Part model, mm, in its own coordinate system. A direction names the side the tool comes from. Coordinates: 2 decimals unless noted, no trailing zeros. One line per question, with ' | ' between items. Start each with the question number.
from build123d import *

# Parameters (mm, degrees)
F0_R            = 45
F0_R_2          = 12.5
F1_DEPTH        = 5
F3_DEPTH        = 10.001
F3_COPIES_COUNT = 8
F4_SIZE         = 0.5
F5_R            = 2


# Not quite as in the source:
# - a pattern or mirror of a feature is missing from the dataset's text; its kind, count and spacing are read off the source's solid


with BuildPart() as f1:
    # F0 (on Front) → F1 (new body, symmetric)
    with BuildSketch(Plane.XZ):
        Circle(F0_R)
        Circle(F0_R_2, mode=Mode.SUBTRACT)
    extrude(amount=F1_DEPTH, both=True)

    # F2 (on face) → F3 (cut, through all)
    with BuildSketch(Plane.XZ.offset(5)):
        Polygon((3.36, 28.75), (0, 33.55), (-3.36, 28.75), (0, 23.95), align=None)
    f3 = extrude(amount=-F3_DEPTH, mode=Mode.SUBTRACT)

    # F3_copies: F3 ×8 about axis
    f3_copies_axis = Axis((0, 0, 0), (0, 1, 0))
    for i in range(1, F3_COPIES_COUNT):
        add(f3.rotate(f3_copies_axis, i * 360 / F3_COPIES_COUNT), mode=Mode.SUBTRACT)

    # F4
    f4_edges = [f1.edges().sort_by_distance(p)[0] for p in [
        (1.68, -5, 31.15),
        (-1.68, -5, 31.15),
        (-1.68, -5, 26.35),
        (1.68, -5, 26.35),
        (1.68, 5, 31.15),
        (-1.68, 5, 31.15),
        (-1.68, 5, 26.35),
        (1.68, 5, 26.35),
        (-23.214316, 5, -20.838437),
        (-19.820203, 5, -17.444324),
        (-20.838437, 5, -23.214316),
        (-17.444324, 5, -19.820203),
        (-31.15, 5, 1.68),
        (-26.35, 5, 1.68),
        (-31.15, 5, -1.68),
        (-26.35, 5, -1.68),
        (-1.68, 5, -31.15),
        (-1.68, 5, -26.35),
        (1.68, 5, -31.15),
        (1.68, 5, -26.35),
        (20.838437, 5, -23.214316),
        (17.444324, 5, -19.820203),
        (23.214316, 5, -20.838437),
        (19.820203, 5, -17.444324),
        (-20.838437, 5, 23.214316),
        (-23.214316, 5, 20.838437),
        (-19.820203, 5, 17.444324),
        (-17.444324, 5, 19.820203),
        (31.15, 5, -1.68),
        (26.35, 5, -1.68),
        (31.15, 5, 1.68),
        (26.35, 5, 1.68),
        (23.214316, 5, 20.838437),
        (19.820203, 5, 17.444324),
        (20.838437, 5, 23.214316),
        (17.444324, 5, 19.820203),
        (-23.214316, -5, -20.838437),
        (-19.820203, -5, -17.444324),
        (-20.838437, -5, -23.214316),
        (-17.444324, -5, -19.820203),
        (-31.15, -5, 1.68),
        (-26.35, -5, 1.68),
        (-31.15, -5, -1.68),
        (-26.35, -5, -1.68),
        (-1.68, -5, -31.15),
        (-1.68, -5, -26.35),
        (1.68, -5, -31.15),
        (1.68, -5, -26.35),
        (20.838437, -5, -23.214316),
        (17.444324, -5, -19.820203),
        (23.214316, -5, -20.838437),
        (19.820203, -5, -17.444324),
        (-20.838437, -5, 23.214316),
        (-23.214316, -5, 20.838437),
        (-19.820203, -5, 17.444324),
        (-17.444324, -5, 19.820203),
        (31.15, -5, -1.68),
        (26.35, -5, -1.68),
        (31.15, -5, 1.68),
        (26.35, -5, 1.68),
        (23.214316, -5, 20.838437),
        (19.820203, -5, 17.444324),
        (20.838437, -5, 23.214316),
        (17.444324, -5, 19.820203),
    ]]
    chamfer(f4_edges, length=F4_SIZE)

    # F5
    f5_edges = [f1.edges().sort_by_distance(p)[0] for p in [
        (-45, -5, 0),
        (-45, 5, 0),
        (-12.5, -5, 0),
        (12.5, 0, 0),
        (-12.5, 5, 0),
    ]]
    fillet(f5_edges, radius=F5_R)


solid = f1.part
1) Tool access for faces 1 (the flat face through (1.75, -4.746, -31.48)), 2 (the flat face through (-26.02, 4.747, 1.75)), 3 (the flat face through (17.45, -0.06, 19.86)): list every direction of +Z, -Z, +X, -X, +Y, -Y with a clear straight run to the whole face (end or side of a thin tool).
2) Band-saw the part on A-A on y = 1. Count the separate pieces of the cut face and the enclosed holes in it, then the cut area to 3 significant figures.
3) Wall check: line 1 along Z through (x, y) = (-19.5, 4); line 2 along X through (y, z) = (3.25, 1.5); line 3 along Z through (x, y) = (-20, 1.5). Give the ranges that are in metal, low to high. Write a range as [from, to].
4) Mould opens along X. For faces 4 (the flat face through (-1, -5, -19)), 5 (the flat face through (31.48, 4.746, 1.75)) say: +X half, -X half, draft (parallel to the pull), parting line (faces both ways), or undercut.
5) Pin check, flat tips, straight feed: pin 1 Ø6 at (y, z) = (2, 17.5) entering from +X; pin 2 Ø6 at (y, z) = (3, 27.5) entering from -X; pin 3 Ø4 at (y, z) = (0, 20.5) entering from -X. Stop position of each tip, or through.
Values found:
1) face 1: -Y | face 2: +Y | face 3: +Y, -Y
2) separate pieces: 1 | enclosed holes: 9 | area: 5,610 mm²
3) line 1: [-40.26, -22.98], [-17.39, 17.39], [22.98, 40.26] | line 2: [-44.96, -31.41], [-26.09, -12.43], [12.43, 26.09], [31.41, 44.96] | line 3: [-40.31, -23.07], [-17.48, 17.48], [23.07, 40.31]
4) face 4: draft | face 5: undercut
5) pin 1: x = 42.6 | pin 2: x = -37.75 | pin 3: x = -41.02
